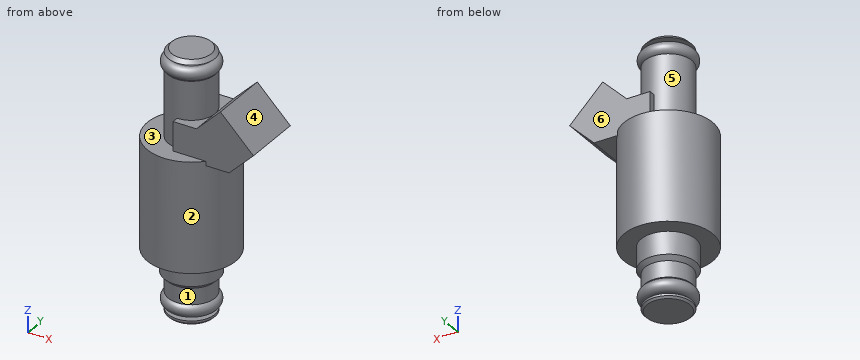
```python
from build123d import *

# Parameters (mm, degrees)
F3_DEPTH = 8.3058


with BuildPart() as f1:
    # F0 (on Front) → F1 (revolve)
    with BuildSketch(Plane.XZ):
        with BuildLine():
            Line((5.4849602437, 72.39), (0, 72.39))
            Line((0, 72.39), (0, 0))
            Line((0, 0), (5.9791589156, 0))
            Line((5.9791589156, 0), (6.5, 0.5208410844))
            Line((6.5, 0.5208410844), (6.5, 1.1235540733))
            Line((6.5, 1.1235540733), (3.81, 1.1235540733))
            Line((3.81, 1.1235540733), (3.81, 1.958))
            Line((3.81, 1.958), (5.625, 1.958))
            ThreePointArc((5.625, 1.958), (7.44, 3.773), (5.625, 5.588))
            Line((5.625, 5.588), (6.5, 5.588))
            Line((6.5, 5.588), (6.5, 10.1114138961))
            Line((6.5, 10.1114138961), (7.62, 11.2314138961))
            Line((7.62, 11.2314138961), (7.62, 17.5331309438))
            Line((7.62, 17.5331309438), (12.319, 17.5331309438))
            Line((12.319, 17.5331309438), (12.319, 48.1258220971))
            Line((12.319, 48.1258220971), (6.5, 48.1258220971))
            Line((6.5, 48.1258220971), (6.5, 66.929))
            Line((6.5, 66.929), (5.625, 66.929))
            ThreePointArc((5.625, 66.929), (7.44, 68.744), (5.625, 70.559))
            Line((5.625, 70.559), (3.81, 70.559))
            Line((3.81, 70.559), (3.81, 71.3749602437))
            Line((3.81, 71.3749602437), (6.5, 71.3749602437))
            Line((6.5, 71.3749602437), (5.4849602437, 72.39))
        make_face()
    revolve(axis=Axis((0, 0, 36.195), (0, 0, -1)))

    # F2 (on Front) → F3 (join, symmetric)
    with BuildSketch(Plane.XZ):
        Polygon((13.188126497, 62.9115402699), (6.5, 56.2234137729), (0, 56.2234137729), (0, 46.9192864976), (12.319, 46.9192864976), (15.6018657007, 46.9192864976), (22.391122985, 53.7085437818), align=None)
    extrude(amount=F3_DEPTH, both=True)


solid = f1.part
```
Could you check a few things on this model? Use its own coordinates, in mm. Face numbers are marked on the shaded views. A direction names the side the tool comes from. Round coordinates to 2 decimals unless told otherwise and drop trailing zeros. Order: outer loops, then holes, each group sorted by start corner. A loop starts at its lowest first (then second) coordinate and runs counter-clockwise, first axis right, second up. Notation, with made-up numbers: M 80.5,8 L 93.5,8 A22 cw 93.5,36 Z; hole C -37.5,66.5 d6. An arc over 180 degrees is marked long. One line per question, with ' | ' between items. Start each with the question number.
(1) Thinking about a two-plate mould opening in X: for the marked faces 4, 5 and 6, which applies, +X half, -X half, draft (parallel to the pull), parting line (faces both ways), or undercut?
(2) Suppose I cut it at D-D on x = 19.5. List the corners of the cut face in (y, z) for me, then the cut area to 3 significant figures.
(3) For P1, Ø10.5, axis at x = 1.5, y = -2.5, coming from the -Z side; P2, Ø5, axis at x = 9, z = 55.5, coming from the -Y side; P3, Ø6, axis at x = -6, y = -7.5, coming from the -Z side; P4, Ø3, axis at y = -1, z = 30, coming from the +X side, each with a flat end and sliding along its axis, tell me the tip position at first contact or that it passes through.
(4) Suppose I cut it at A-A on x = 10. List the corners of the cut face in (y, z) for me, then the cut area to 3 significant figures.
(5) For the marked faces 1, 2 and 3, which set-ups out of +Z, -Z, +X, -X, +Y, -Y let a thin tool reach every point of the face, with its end or its side?
(6) Please list where these lines run through material, in increasing order: line 1 along Z through (x, y) = (7, -1.25); line 2 along Z through (x, y) = (-11, 3); line 3 along X through (y, z) = (-0.5, 44).
(7) Suppose I cut it at B-B on z = 55. List the corners of the cut face in (x, y) for me.
(8) Suppose I cut it at C-C on z = 30.5. List the corners of the cut face in (x, y) for me.
Geometry results:
1) face 4: +X half | face 5: undercut | face 6: draft
2) outline: M -8.31,50.82 L 8.31,50.82 L 8.31,56.6 L -8.31,56.6 Z | area: 96.1 mm²
3) P1: z = 0 | P2: y = -8.31 | P3: z = 2.25 | P4: x = 12.32
4) outline: M -8.31,46.92 L -7.19,46.92 L -7.19,17.53 L 7.19,17.53 L 7.19,46.92 L 8.31,46.92 L 8.31,59.72 L -8.31,59.72 Z | area: 636 mm²
5) face 1: none | face 2: -Z | face 3: -X
6) line 1: 2.73 to 4.82, 10.72 to 56.72, 67.7 to 69.79 | line 2: 17.53 to 48.13 | line 3: -12.31 to 12.31
7) outline: M 0,-8.31 L 21.1,-8.31 L 21.1,8.31 L 0,8.31 L 0,6.5 A6.5 ccw 0,-6.5 Z
8) outline: C 0,0 d24.64
